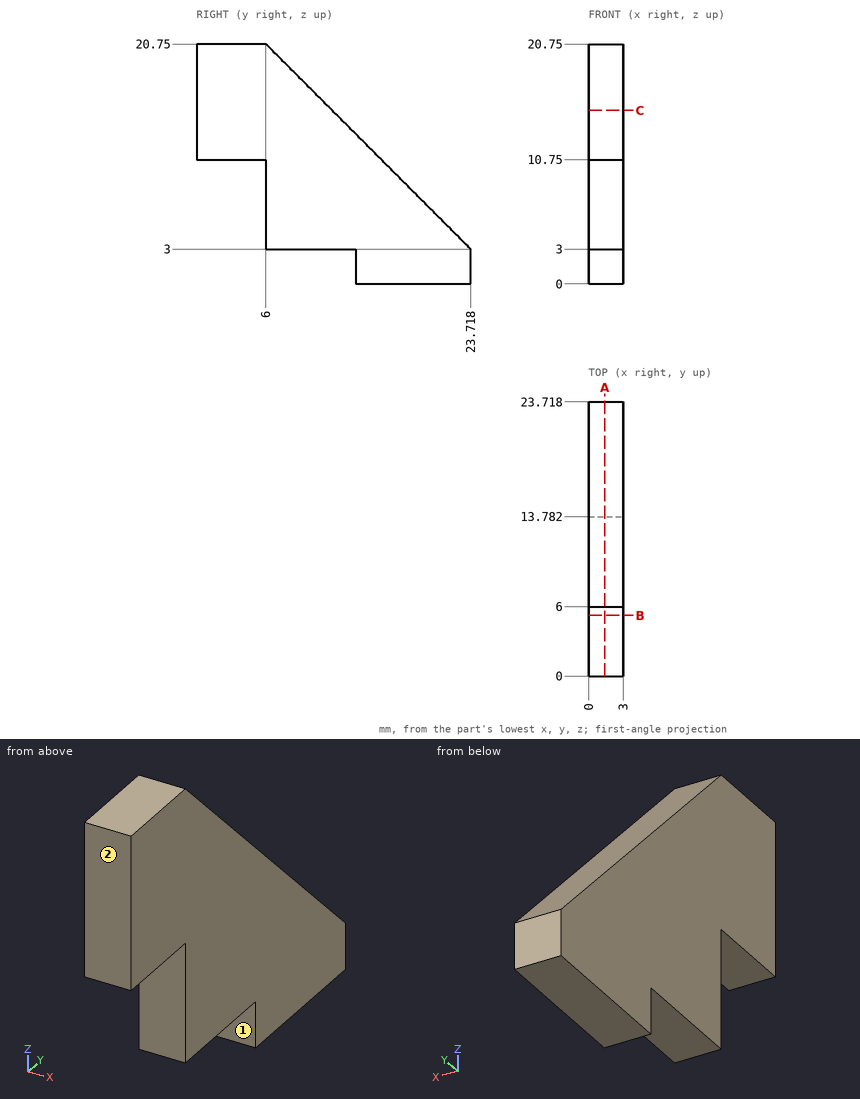
Geometry: see drawing. Coordinates: mm, zero at the bounding-box minimum. A direction names the side the tool comes from. Round coordinates to 2 decimals unless told otherwise and drop trailing zeros. Order: outer loops, then holes, each group sorted by start corner. A loop starts at its lowest first (then second) coordinate and runs counter-clockwise, first axis right, second up. Notation, with made-up numbers: (8.5, 64.5) - (59.5, 64.5) arc R23 cw to (59.5, 81.5) - close; hole circle Ø8 at (40, -26.5). An arc over 180 degrees is marked (long way). Use a Markdown table: item, result. Add a question column.
1. Line query: probe 1 along Y at (x, z) = (0.9, 1.75); probe 2 along Z at (x, y) = (2.05, 1.5); probe 3 along Z at (x, y) = (1.4, 13). Output: solid intervals per line, ascending.
2. Section query A-A (x = 1.4). Return the cut outline in (y, z), then the cut area to 3 significant figures.
3. Set-up query: the marked faces 1 and 2. Return all of +Z, -Z, +X, -X, +Y, -Y with unobstructed straight access to the full face (end or side cutting, diameter ignored); none if empty.
4. First-contact query: pin 1 (1.5 mm diameter, centred on x = 2, z = 1.5, fed in from -Y); pin 2 (1.5 mm diameter, centred on x = 1, y = 9.5, fed in from -Z); pin 3 (0.9 mm diameter, centred on x = 1, z = 6.5, fed in from -Y). Flat tips, straight axial feed; report the tip coordinate or a pass-through.
5. Section query B-B (y = 5.25). Return the cut outline in (x, z), then the cut area to 3 significant figures.
6. Section query C-C (z = 15). Return the cut outline in (x, y), then the cut area to 3 significant figures.
Derived:
| question | item | result |
|---|---|---|
| 1 | probe 1 | 13.78 to 23.72 |
| 1 | probe 2 | 10.75 to 20.75 |
| 1 | probe 3 | 3 to 13.74 |
| 2 | outline | (0, 10.75) - (6, 10.75) - (6, 3) - (13.78, 3) - (13.78, 0) - (23.72, 0) - (23.72, 3) - (6, 20.75) - (0, 20.75) - close |
| 2 | area | 247 mm2 |
| 3 | face 1 | -Z, +X, -X, -Y |
| 3 | face 2 | +Z, -Z, +X, -X, -Y |
| 4 | pin 1 | y = 13.78 |
| 4 | pin 2 | z = 3 |
| 4 | pin 3 | y = 6 |
| 5 | outline | (0, 10.75) - (3, 10.75) - (3, 20.75) - (0, 20.75) - close |
| 5 | area | 30.0 mm2 |
| 6 | outline | (0, 0) - (3, 0) - (3, 11.74) - (0, 11.74) - close |
| 6 | area | 35.2 mm2 |
